Work out the finished part from the listing and answer in its coordinate system (mm). Round coordinates to 2 decimals unless told otherwise and drop trailing zeros. Loops run counter-clockwise (first coordinate to the right, second up) from the corner with the lowest first, then second, coordinate; pieces in that order, holes last. Notation, with made-up numbers: M -26.75,74 L -11.75,74 A29 ccw -11.75,95 Z; hole C -8,-26 d7. An arc over 180 degrees is marked long. One line per item, written item: value.
```python
from build123d import *

# Parameters (mm, degrees)
SKETCH1_R                    = 15
BOSS_EXTRUDE1_DEPTH          = 17.5
SKETCH2_OUTSIDE_W            = 192.554
SKETCH2_OUTSIDE_H            = 200.592
SKETCH2_OUTSIDE_R            = 25.980762114
CUT_EXTRUDE1_DEPTH           = 17.5
CUT_EXTRUDE1_TAPER           = 60
CUT_EXTRUDE1_OTHER_WAY_DEPTH = 17.5
CUT_EXTRUDE1_OTHER_WAY_DRAFT = -60
MIRROR1_COPY_1_SKETCH_W      = 192.554
MIRROR1_COPY_1_SKETCH_H      = 200.592
MIRROR1_COPY_1_SKETCH_R      = 25.980762114
MIRROR1_COPY_1_DEPTH         = 17.5
MIRROR1_COPY_1_DRAFT         = -60
MIRROR1_COPY_2_SKETCH_W      = 192.554
MIRROR1_COPY_2_SKETCH_H      = 200.592
MIRROR1_COPY_2_SKETCH_R      = 25.980762114
MIRROR1_COPY_2_DEPTH         = 17.5
MIRROR1_COPY_2_DRAFT         = -60


with BuildPart() as part:
    # Sketch1 → Boss-Extrude1 (new, symmetric)
    with BuildSketch(Plane(origin=(0, 0, 0), x_dir=(1, 0, 0), z_dir=(0, 1, 0))):
        Polygon((0, 30), (-25.980762114, 15), (-25.980762114, -15), (0, -30), (25.980762114, -15), (25.980762114, 15), align=None)
        with Locations(Location((0, 0, 0), (0, 0, 270))):
            Circle(SKETCH1_R, mode=Mode.SUBTRACT)
    extrude(amount=BOSS_EXTRUDE1_DEPTH, both=True)

    # Sketch2 outside → Cut-Extrude1 (cut)
    with BuildSketch(Plane(origin=(0, 17.5, 0), x_dir=(1, 0, 0), z_dir=(0, 1, 0))):
        Rectangle(SKETCH2_OUTSIDE_W, SKETCH2_OUTSIDE_H)
        Circle(SKETCH2_OUTSIDE_R, mode=Mode.SUBTRACT)
    cut_extrude1 = extrude(amount=CUT_EXTRUDE1_DEPTH, taper=CUT_EXTRUDE1_TAPER, mode=Mode.SUBTRACT)


with BuildPart() as cut_extrude1_other_way_tool:
    # Sketch2 outside → Cut-Extrude1 other way (with draft: the straight prism first)
    with BuildSketch(Plane(origin=(0, 17.5, 0), x_dir=(1, 0, 0), z_dir=(0, 1, 0))):
        Rectangle(SKETCH2_OUTSIDE_W, SKETCH2_OUTSIDE_H)
        Circle(SKETCH2_OUTSIDE_R, mode=Mode.SUBTRACT)
    extrude(amount=-CUT_EXTRUDE1_OTHER_WAY_DEPTH)
    # Cut-Extrude1 other way: the draft: its side faces are tilted about the plane it starts from
    cut_extrude1_other_way_sides = [cut_extrude1_other_way_tool.faces().sort_by_distance(p)[0] for p in [
        (0, 8.75, 100.296),
        (96.277, 8.75, 0),
        (0, 8.75, -100.296),
        (-96.277, 8.75, 0),
        (-25.980762114, 8.75, 0),
    ]]
    draft(cut_extrude1_other_way_sides, Plane(origin=(0, 17.5, 0), x_dir=(1, 0, 0), z_dir=(0, 1, 0)), CUT_EXTRUDE1_OTHER_WAY_DRAFT)


with BuildPart() as part_1:
    add(part.part)

    # Cut-Extrude1 other way: cut by cut_extrude1_other_way_tool
    add(cut_extrude1_other_way_tool.part, mode=Mode.SUBTRACT)

    # Mirror1: Cut-Extrude1 across plane
    add(cut_extrude1.mirror(Plane.ZX), mode=Mode.SUBTRACT)


with BuildPart() as mirror1_copy_1_tool:
    # Mirror1 copy 1 sketch → Mirror1 copy 1 (with draft: the straight prism first)
    with BuildSketch(Plane.XZ.offset(17.5)):
        Rectangle(MIRROR1_COPY_1_SKETCH_W, MIRROR1_COPY_1_SKETCH_H)
        Circle(MIRROR1_COPY_1_SKETCH_R, mode=Mode.SUBTRACT)
    extrude(amount=-MIRROR1_COPY_1_DEPTH)
    # Mirror1 copy 1: the draft: its side faces are tilted about the plane it starts from
    mirror1_copy_1_sides = [mirror1_copy_1_tool.faces().sort_by_distance(p)[0] for p in [
        (0, -8.75, 100.296),
        (96.277, -8.75, 0),
        (0, -8.75, -100.296),
        (-96.277, -8.75, 0),
        (-25.980762114, -8.75, 0),
    ]]
    draft(mirror1_copy_1_sides, Plane.XZ.offset(17.5), MIRROR1_COPY_1_DRAFT)


with BuildPart() as part_2:
    add(part_1.part)

    # Mirror1 copy 1: cut by mirror1_copy_1_tool
    add(mirror1_copy_1_tool.part, mode=Mode.SUBTRACT)


with BuildPart() as mirror1_copy_2_tool:
    # Mirror1 copy 2 sketch → Mirror1 copy 2 (with draft: the straight prism first)
    with BuildSketch(Plane.XZ.offset(17.5)):
        Rectangle(MIRROR1_COPY_2_SKETCH_W, MIRROR1_COPY_2_SKETCH_H)
        Circle(MIRROR1_COPY_2_SKETCH_R, mode=Mode.SUBTRACT)
    extrude(amount=-MIRROR1_COPY_2_DEPTH)
    # Mirror1 copy 2: the draft: its side faces are tilted about the plane it starts from
    mirror1_copy_2_sides = [mirror1_copy_2_tool.faces().sort_by_distance(p)[0] for p in [
        (0, -8.75, 100.296),
        (96.277, -8.75, 0),
        (0, -8.75, -100.296),
        (-96.277, -8.75, 0),
        (-25.980762114, -8.75, 0),
    ]]
    draft(mirror1_copy_2_sides, Plane.XZ.offset(17.5), MIRROR1_COPY_2_DRAFT)


with BuildPart() as part_3:
    add(part_2.part)

    # Mirror1 copy 2: cut by mirror1_copy_2_tool
    add(mirror1_copy_2_tool.part, mode=Mode.SUBTRACT)


solid = part_3.part
```
1) Find section A-A (y = -9.5). Give the vertices of the cut face in (x, z).
Check values:
outline: M -25.98,-15 L 0,-30 L 25.98,-15 L 25.98,15 L 0,30 L -25.98,15 Z; hole C 0,0 d30
2) Find the intervals of material crossed by probe 1 along X at (y, z) = (9.5, 0); probe 2 along X at (y, z) = (13.5, -13); probe 3 along Z at (x, y) = (1, -7.5), in increasing order. Write a range as from..to.
Check values:
probe 1: -25.98..-15, 15..25.98
probe 2: -25.98..-7.48, 7.48..25.98
probe 3: -29.42..-14.97, 14.97..29.42
3) The mould has two halves that part along X. Classify faces 1 (the face through (0.66, -0.245, -14.985)), 2 (the face through (-23.36, -16.95, -13.41)), 3 (the face through (25.981, 0, 0)): +X half, -X half, draft (parallel to the pull), parting line (faces both ways), or undercut.
Check values:
face 1: undercut
face 2: -X half
face 3: +X half
4) Each of these flat-tipped pins is pushed along its axis until it touches: pin 1 (3 mm diameter, centred on x = -10, y = 8.5, fed in from -Z); pin 2 (1 mm diameter, centred on y = 0, z = 23.5, fed in from +X); pin 3 (8 mm diameter, centred on x = -10, y = -1.5, fed in from +Z); pin 4 (18 mm diameter, centred on x = 0, z = 0, fed in from +Y). Where does it stop, or does it pass through?
Check values:
pin 1: z = -25.09
pin 2: x = 12.12
pin 3: z = 26.54
pin 4: through
